Design review of the part built by this model. Coordinates are the model's own, in mm. A direction names the side the tool comes from. Round coordinates to 2 decimals unless told otherwise and drop trailing zeros. Loops run counter-clockwise (first coordinate to the right, second up) from the corner with the lowest first, then second, coordinate; pieces in that order, holes last. Notation, with made-up numbers: (2.25, 33) - (43.25, 33) arc R21 cw to (43.25, 39) - close; hole circle Ø11 at (42.5, 40.25). An arc over 180 degrees is marked (long way). Return JSON: item names as keys, results as strings. Group by question number.
from build123d import *

# Parameters (mm, degrees)
SKETCH_1_W          = 56.4
SKETCH_1_H          = 56.4
EXTRUDE_1_DEPTH     = 53
SKETCH_2_R          = 20
EXTRUDE_2_DEPTH     = 2.5
SKETCH_3_R          = 7
EXTRUDE_3_DEPTH     = 31.5
FILLET_1_R          = 5
SKETCH_4_R          = 2.6
CUT_EXTRUDE_1_DEPTH = 54


with BuildPart() as part:
    # 草图1 → 凸台-拉伸1 (new body)
    with BuildSketch(Plane.XY):
        with Locations((28.2, 28.2)):
            Rectangle(SKETCH_1_W, SKETCH_1_H)
    extrude(amount=EXTRUDE_1_DEPTH)

    # 草图2 → 凸台-拉伸2 (add)
    with BuildSketch(Plane.XY.offset(53)):
        with Locations((28.2, 28.2)):
            Circle(SKETCH_2_R)
    extrude(amount=EXTRUDE_2_DEPTH)

    # 草图3 → 凸台-拉伸3 (add)
    with BuildSketch(Plane.XY.offset(55.5)):
        with Locations((28.2, 28.2)):
            Circle(SKETCH_3_R)
    extrude(amount=EXTRUDE_3_DEPTH)

    # 圆角1
    fillet_1_edges = [part.edges().sort_by_distance(p)[0] for p in [
        (0, 56.4, 26.5),
        (56.4, 56.4, 26.5),
        (56.4, 0, 26.5),
        (0, 0, 26.5),
    ]]
    fillet(fillet_1_edges, radius=FILLET_1_R)

    # 草图4 → 切除-拉伸1 (cut, through all)
    with BuildSketch(Plane.XY.offset(53)):
        with Locations((4.615, 51.785)):
            Circle(SKETCH_4_R)
        with Locations((51.785, 51.785)):
            Circle(SKETCH_4_R)
        with Locations((51.785, 4.615)):
            Circle(SKETCH_4_R)
        with Locations((4.615, 4.615)):
            Circle(SKETCH_4_R)
    extrude(amount=-CUT_EXTRUDE_1_DEPTH, mode=Mode.SUBTRACT)


solid = part.part
Q1. Add section C-C, the plane z = 64. State the section outline as (x, y) points.
Q2. Add section D-D, the plane y = 46.5. State the section outline as (x, z) points.
Q3. Tool access review of faces 1 (the flat face through (28, 29, 0)), 2 (the flat face through (21.5, 47.4, 53)): name each direction out of +Z, -Z, +X, -X, +Y, -Y from which nothing blocks a thin tool from reaching the whole face with its end or side.
Q4. For line 1 (X direction, y = 53, z = 6); line 2 (X direction, y = 4.5, z = 46); line 3 (Z direction, x = 20.5, y = 23), list the stretches that pass through material, from the lowest coordinate up.
Q5. Draft analysis for pull direction X (two halves, no side actions). For faces 3 (the cylindrical face through (49.188, 4.729, 26.871)), 4 (the cylindrical face through (49.722, 50.203, 26.871)), 5 (the cylindrical face through (54.9, 54.97, 26.87)), 6 (the cylindrical face through (23.04, 32.93, 71.03)), state which applies: pulls with the +X half, pulls with the -X half, needs draft (parallel to the pull), parting line crosses it, or undercut.
Q6. Add section A-A, the plane x = 28.2. State the section outline as (y, z) points, plus the area to 3 significant figures.
Q7. Insertion check: pin 1 Ø2 at (x, z) = (17.5, 55.5) entering from -Y; pin 2 Ø7 at (x, y) = (4.615, 4.615) entering from +Z; pin 3 Ø1.5 at (x, z) = (10.5, 54) entering from -Y. Each pin has a flat end and moves straight along its axis. Give the tip position at first contact, or say it passes through.
Evaluation:
{
 "1": {"outline": "circle Ø14 at (28.2, 28.2)"},
 "2": {"outline": "(0, 0) - (56.4, 0) - (56.4, 53) - (36.27, 53) - (36.27, 55.5) - (20.13, 55.5) - (20.13, 53) - (0, 53) - close"},
 "3": {"face 1": "-Z, +X, -X, +Y, -Y", "face 2": "+Z"},
 "4": {"line 1": "0.26 to 2.32, 6.91 to 49.49, 54.08 to 56.14", "line 2": "0.03 to 2.02, 7.21 to 49.19, 54.38 to 56.37", "line 3": "0 to 55.5"},
 "5": {"face 3": "undercut", "face 4": "undercut", "face 5": "pulls with the +X half", "face 6": "parting line crosses it"},
 "6": {"outline": "(0, 0) - (56.4, 0) - (56.4, 53) - (48.2, 53) - (48.2, 55.5) - (35.2, 55.5) - (35.2, 87) - (21.2, 87) - (21.2, 55.5) - (8.2, 55.5) - (8.2, 53) - (0, 53) - close", "area": "3,530 mm²"},
 "7": {"pin 1": "y = 10.71", "pin 2": "z = 53", "pin 3": "y = 17.58"}
}
